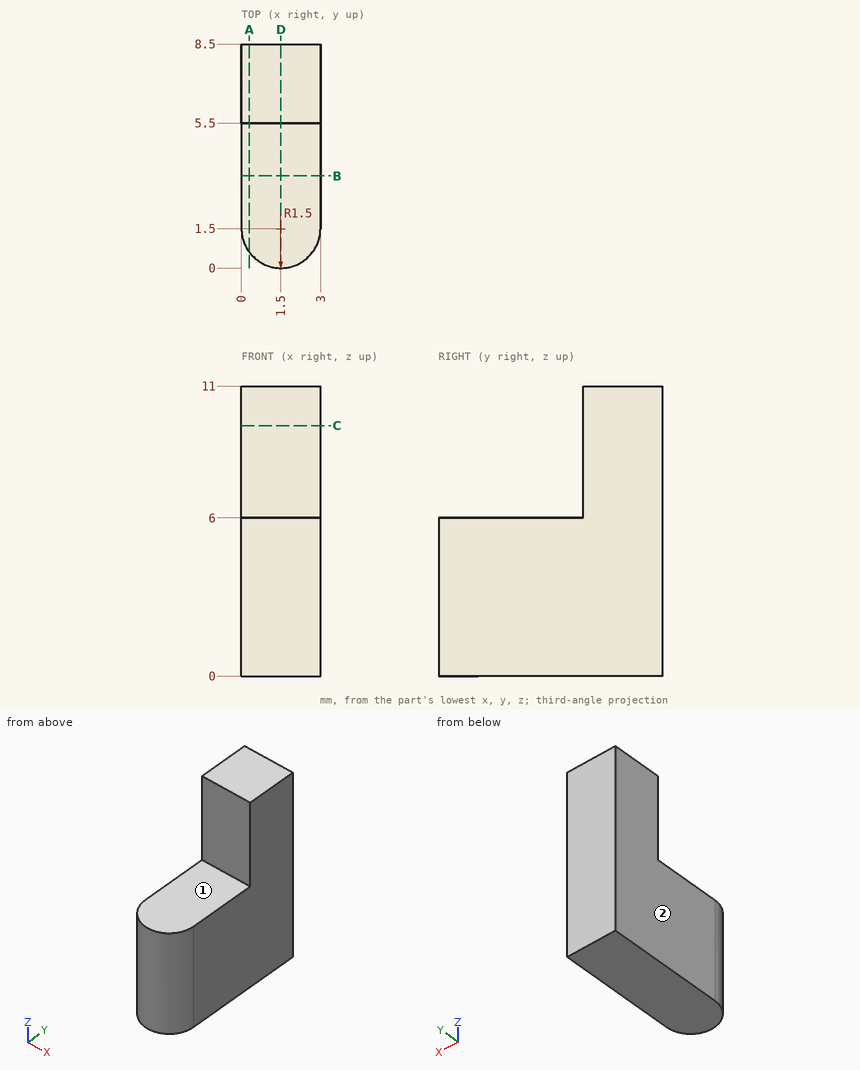
Verification items for this drawing (mm, ordinates from the low corner). A direction names the side the tool comes from. Coordinates: 2 decimals unless noted, no trailing zeros. Order: outer loops, then holes, each group sorted by start corner. A loop starts at its lowest first (then second) coordinate and runs counter-clockwise, first axis right, second up. Notation, with made-up numbers: (27, 87) - (36, 87) arc R25 cw to (36, 110) - close; hole circle Ø11 at (-13, 41.5). An arc over 180 degrees is marked (long way). Answer as a JSON object with one key per item and string values. Group by question number.
Item 1: Sectioned sample at A-A, the plane x = 0.3. Record the cut outline in (y, z), and give its area (3 significant figures).
Item 2: Tool access check on the marked faces 1 and 2. Record the directions out of +Z, -Z, +X, -X, +Y, -Y that give a thin tool (end or side, any length) a straight path to the whole face; none if there is none.
Item 3: Sectioned sample at C-C, the plane z = 9.5. Record the cut outline in (x, y), and give its area (3 significant figures).
Item 4: Scan lines: probe 1 along Z at (x, y) = (0.75, 4.5); probe 2 along Y at (x, z) = (1.4, 7.75); probe 3 along Y at (x, z) = (1.1, 5.25). Record each from-to range of solid material in increasing order.
Item 5: Sectioned sample at D-D, the plane x = 1.5. Record the cut outline in (y, z), and give its area (3 significant figures).
Item 6: Depth check by flat-ended pin: pin 1 Ø1.5 at (x, z) = (1, 7.5) entering from -Y. Enter the tip coordinate at first touch or a pass-through.
Item 7: Sectioned sample at B-B, the plane y = 3.5. Record the cut outline in (x, z), and give its area (3 significant figures).
Resolved:
{
 "1": {"outline": "(0.6, 0) - (8.5, 0) - (8.5, 11) - (5.5, 11) - (5.5, 6) - (0.6, 6) - close", "area": "62.4 mm^2"},
 "2": {"face 1": "+Z, +X, -X, -Y", "face 2": "+Z, -Z, -X, +Y, -Y"},
 "3": {"outline": "(0, 5.5) - (3, 5.5) - (3, 8.5) - (0, 8.5) - close", "area": "9.00 mm^2"},
 "4": {"probe 1": "0 to 6", "probe 2": "5.5 to 8.5", "probe 3": "0.05 to 8.5"},
 "5": {"outline": "(0, 0) - (8.5, 0) - (8.5, 11) - (5.5, 11) - (5.5, 6) - (0, 6) - close", "area": "66.0 mm^2"},
 "6": {"pin 1": "y = 5.5"},
 "7": {"outline": "(0, 0) - (3, 0) - (3, 6) - (0, 6) - close", "area": "18.0 mm^2"}
}
